```python
from build123d import *

# Parameters (mm, degrees)
BOSS_EXTRUDE1_DEPTH   = 60
BOSS_EXTRUDE1_2_DEPTH = 60
SKETCH3_W             = 219
SKETCH3_H             = 10
BOSS_EXTRUDE3_DEPTH   = 20


with BuildPart() as part:
    # Sketch1 → Boss-Extrude1 (new body)
    with BuildSketch(Plane(origin=(0, 0, 0), x_dir=(1, 0, 0), z_dir=(0, 1, 0))):
        Polygon((-109.5, 12.700803213), (-109.5, -87.299196787), (-27.5, 12.700803213), (-27.5, 42.700803213), (-109.5, 42.700803213), align=None)
        Polygon((-94.5, 27.700803213), (-94.5, -45.350177528), (-42.5, 12.700803213), (-42.5, 27.700803213), align=None, mode=Mode.SUBTRACT)
    extrude(amount=BOSS_EXTRUDE1_DEPTH)



with BuildPart() as body_2:
    # Sketch1 → Boss-Extrude1 2 (new body)
    with BuildSketch(Plane(origin=(0, 0, 0), x_dir=(1, 0, 0), z_dir=(0, 1, 0))):
        Polygon((109.5, 42.700803213), (27.5, 42.700803213), (27.5, 12.700803213), (109.5, -87.299196787), (109.5, 12.700803213), align=None)
        Polygon((42.5, 12.700803213), (42.5, 27.700803213), (94.5, 27.700803213), (94.5, -45.350177528), align=None, mode=Mode.SUBTRACT)
    extrude(amount=BOSS_EXTRUDE1_2_DEPTH)


with BuildPart() as part_1:
    add(part.part)

    add(body_2.part)  # Boss-Extrude3 merges body 2
    # Sketch3 → Boss-Extrude3 (add)
    with BuildSketch(Plane(origin=(0, 60, 0), x_dir=(1, 0, 0), z_dir=(0, 1, 0))):
        with Locations((0, 37.700803213)):
            Rectangle(SKETCH3_W, SKETCH3_H)
    extrude(amount=BOSS_EXTRUDE3_DEPTH)


solid = part_1.part
```
Here's how the part is built. I have some questions about the finished solid (model axes, mm). A direction names the side the tool comes from. Give positions to 0.01 mm unless a question says otherwise; leave off trailing zeros. Loops run counter-clockwise (first coordinate to the right, second up) from the corner with the lowest first, then second, coordinate; pieces in that order, holes last. Notation, with made-up numbers: (42.25, -10) -> (66.25, -10) arc R22 cw to (66.25, 13) -> close; hole circle Ø7 at (87.5, 54). An arc over 180 degrees is marked (long way). Use one line per item in the form item = value. Start each with the question number.
1) Imagine slicing it at A-A (y = 40.5). Please give me the cut outline in (x, z).
2) Imagine slicing it at B-B (x = -67.5). Please give me the cut outline in (y, z), then the cut area to 3 significant figures.
3) Which directions (+Z, -Z, +X, -X, +Y, -Y) give clear straight access to the entire face, cutting with the end or side of a thin tool? Please do faces 1 (the face through (94.5, 30, 8)), 2 (the face through (-27.5, 30, -27)), 3 (the face through (-69.074, 29.58, 37.999)), 4 (the face through (-96, 60, 13)).
4) Imagine slicing it at D-D (z = 39). Please give me the cut outline in (x, y), then the cut area to 3 significant figures.
5) For P1, Ø5, axis at x = -24.5, y = 24, coming from the -Z side; P2, Ø6, axis at x = -40.5, y = 71, coming from the +Z side; P3, Ø6, axis at x = 71.5, y = 53, coming from the +Z side; P4, Ø11, axis at x = -10.5, z = -37.5, coming from the -Y side, each with a flat end and sliding along its axis, tell me the tip position at first contact or that it passes through.
6) Please list where these lines run through material, in increasing order: line 1 along X through (y, z) = (57, 0); line 2 along X through (y, z) = (48.5, 19.5); line 3 along Z through (x, y) = (-78, 64).
7) Imagine slicing it at C-C (z = 67). Please give me the cut outline in (x, y).
8) Thinking about a two-plate mould opening in X: for faces 5 (the face through (-96, 0, 7)), 6 (the face through (109.5, 31, 23)), 7 (the face through (-42.5, 30, -20)), which applies, +X half, -X half, draft (parallel to the pull), parting line (faces both ways), or undercut?
Check values:
q1.outline = (-109.5, -42.7) -> (-27.5, -42.7) -> (-27.5, -12.7) -> (-109.5, 87.3) -> close; (27.5, -42.7) -> (109.5, -42.7) -> (109.5, 87.3) -> (27.5, -12.7) -> close; hole (-94.5, -27.7) -> (-42.5, -27.7) -> (-42.5, -12.7) -> (-94.5, 45.35) -> close; hole (42.5, -27.7) -> (94.5, -27.7) -> (94.5, 45.35) -> (42.5, -12.7) -> close
q2.outline = (0, -42.7) -> (80, -42.7) -> (80, -32.7) -> (60, -32.7) -> (60, -27.7) -> (0, -27.7) -> close; (0, 15.21) -> (60, 15.21) -> (60, 36.08) -> (0, 36.08) -> close
q2.area = 2,350 mm^2
q3.face_1 = +Y, -Y
q3.face_2 = +Z, -Z, -Y
q3.face_3 = +Z, +Y, -Y
q3.face_4 = +Z, +X, -X, +Y
q4.outline = (-109.5, 0) -> (-94.5, 0) -> (-94.5, 60) -> (-109.5, 60) -> close; (-88.81, 0) -> (-69.89, 0) -> (-69.89, 60) -> (-88.81, 60) -> close; (69.89, 0) -> (88.81, 0) -> (88.81, 60) -> (69.89, 60) -> close; (94.5, 0) -> (109.5, 0) -> (109.5, 60) -> (94.5, 60) -> close
q4.area = 4,070 mm^2
q5.P1 = through
q5.P2 = -32.7
q5.P3 = 44.62
q5.P4 = 60
q6.line_1 = -109.5 to -94.5, -53.88 to -37.91, 37.91 to 53.88, 94.5 to 109.5
q6.line_2 = -109.5 to -94.5, -71.34 to -53.9, 53.9 to 71.34, 94.5 to 109.5
q6.line_3 = -42.7 to -32.7
q7.outline = (-109.5, 0) -> (-92.85, 0) -> (-92.85, 60) -> (-109.5, 60) -> close; (92.85, 0) -> (109.5, 0) -> (109.5, 60) -> (92.85, 60) -> close
q8.face_5 = draft
q8.face_6 = +X half
q8.face_7 = undercut
